Verification items for the finished model (mm, model axes). A direction names the side the tool comes from. Coordinates: 2 decimals unless noted, no trailing zeros. Loops run counter-clockwise (first coordinate to the right, second up) from the corner with the lowest first, then second, coordinate; pieces in that order, holes last.
Q1. Go/stop test with flat-tipped pins: P1, Ø1.5, axis at y = 3, z = 28, coming from the -X side; P2, Ø2.5, axis at x = -109.5, y = 2.5, coming from the +Z side. Record where each tip stops, or that it passes through.
Q2. Access from +Z, -Z, +X, -X, +Y, -Y to the whole of each face (thin tool, end or side, straight path). Record for faces 1 (the face through (98.5, 2, 170)), 2 (the face through (113.5, 2, 26)), 3 (the face through (-113, 2, 158)), 4 (the face through (-118, 2, 21.2)).
Q3. Sectioned sample at A-A (y = 1). Enter the section's corners in (x, z), then the cut area to 3 significant figures.
Q4. Material ranges on probe 1 along X at (y, z) = (3.5, 123.86); probe 2 along X at (y, z) = (4.75, 125), recorded low to high.
Q5. Mould release check, pull along Z, two halves, no side actions. Record for faces 5 (the face through (-98.5, 2, 171)), 6 (the face through (-113.5, 2, 26)), 7 (the face through (114, 2, 158)): +Z half, -Z half, draft (parallel to the pull), parting line (faces both ways), or undercut.
```python
from build123d import *

# Parameters (mm, degrees)
ESQUISSE1_R        = 1.6
BOSS_EXTRU_1_DEPTH = 5


with BuildPart() as part:
    # Esquisse1 → Boss.-Extru.1 (new body)
    with BuildSketch(Plane(origin=(0, 0, 0), x_dir=(1, 0, 0), z_dir=(0, 1, 0))):
        Polygon((-123.5, 5), (123.5, 5), (123.5, -21.2), (113.5, -21.2), (113.5, -31.2), (123.5, -31.2), (123.5, -158), (103.5, -158), (98.5, -163), (98.5, -178), (-98.5, -178), (-98.5, -163), (-103.5, -158), (-123.5, -158), (-123.5, -31.2), (-113.5, -31.2), (-113.5, -21.2), (-123.5, -21.2), align=None)
        with Locations(Location((0, -123.86, 0), (0, 0, 270))):
            Circle(ESQUISSE1_R, mode=Mode.SUBTRACT)
    extrude(amount=BOSS_EXTRU_1_DEPTH)


solid = part.part
```
Geometry check:
1. P1: stops at x = -113.5
1. P2: stops at z = 158
2. face 1: +Z, +X, +Y, -Y
2. face 2: +X, +Y, -Y
2. face 3: +Z, -X, +Y, -Y
2. face 4: -X, +Y, -Y
3. outline: (-123.5, -5) - (123.5, -5) - (123.5, 21.2) - (113.5, 21.2) - (113.5, 31.2) - (123.5, 31.2) - (123.5, 158) - (103.5, 158) - (98.5, 163) - (98.5, 178) - (-98.5, 178) - (-98.5, 163) - (-103.5, 158) - (-123.5, 158) - (-123.5, 31.2) - (-113.5, 31.2) - (-113.5, 21.2) - (-123.5, 21.2) - close; hole circle Ø3.2 at (0, 123.86)
3. area: 44,000 mm2
4. probe 1: x = -123.5 to -1.6, 1.6 to 123.5
4. probe 2: x = -123.5 to -1.12, 1.12 to 123.5
5. face 5: draft
5. face 6: undercut
5. face 7: +Z half
